```python
from build123d import *

# Parameters (mm, degrees)
SKETCH1_R           = 40
BOSS_EXTRUDE1_DEPTH = 100
SKETCH3_R           = 30
BOSS_EXTRUDE2_DEPTH = 180
SKETCH4_R           = 40
BOSS_EXTRUDE3_DEPTH = 100
SKETCH5_W           = 41.242816752
SKETCH5_H           = 81.516639277
CUT_EXTRUDE1_DEPTH  = 80
SKETCH6_W           = 41.962077935
SKETCH6_H           = 81.514478353
CUT_EXTRUDE2_DEPTH  = 80
FILLET3_R           = 40
FILLET4_R           = 40
SKETCH7_R           = 20
BOSS_EXTRUDE4_DEPTH = 10
SKETCH8_R           = 20
BOSS_EXTRUDE5_DEPTH = 10
FILLET5_R           = 40
FILLET6_R           = 40
FILLET7_R           = 10
FILLET8_R           = 10


# Some blends are built 0.0001 mm under size
with BuildPart() as part:
    # Sketch1 → Boss-Extrude1 (new body)
    with BuildSketch(Plane(origin=(0, 0, 0), x_dir=(1, 0, 0), z_dir=(0, 1, 0))):
        with Locations(Location((0, 0, 0), (0, 0, 270))):
            Circle(SKETCH1_R)
    extrude(amount=BOSS_EXTRUDE1_DEPTH)

    # Sketch3 → Boss-Extrude2 (add)
    with BuildSketch(Plane(origin=(0, 100, 0), x_dir=(1, 0, 0), z_dir=(0, 1, 0))):
        with Locations(Location((0, 0, 0), (0, 0, 90))):
            Circle(SKETCH3_R)
    extrude(amount=BOSS_EXTRUDE2_DEPTH)

    # Sketch4 → Boss-Extrude3 (add)
    with BuildSketch(Plane(origin=(0, 280, 0), x_dir=(1, 0, 0), z_dir=(0, 1, 0))):
        with Locations(Location((0, 0, 0), (0, 0, 270))):
            Circle(SKETCH4_R)
    extrude(amount=BOSS_EXTRUDE3_DEPTH)

    # Sketch5 → Cut-Extrude1 (cut)
    with BuildSketch(Plane(origin=(0, 380, 0), x_dir=(1, 0, 0), z_dir=(0, 1, 0))):
        with Locations((20.621408376, 0.242248556)):
            Rectangle(SKETCH5_W, SKETCH5_H)
    extrude(amount=-CUT_EXTRUDE1_DEPTH, mode=Mode.SUBTRACT)

    # Sketch6 → Cut-Extrude2 (cut)
    with BuildSketch(Plane.XZ):
        with Locations((20.981038968, -0.067313451)):
            Rectangle(SKETCH6_W, SKETCH6_H)
    extrude(amount=-CUT_EXTRUDE2_DEPTH, mode=Mode.SUBTRACT)

    # Fillet3
    fillet3_edges = [part.edges().sort_by_distance(p)[0] for p in [
        (-40, 0, 0),
    ]]
    fillet(fillet3_edges, radius=FILLET3_R - 0.0001)  # a hair under: the kernel refuses the full size

    # Fillet4
    fillet4_edges = [part.edges().sort_by_distance(p)[0] for p in [
        (-40, 380, 0),
    ]]
    fillet(fillet4_edges, radius=FILLET4_R - 0.0001)  # a hair under: the kernel refuses the full size

    # Sketch7 → Boss-Extrude4 (add)
    with BuildSketch(Plane(origin=(0, 0, 0), x_dir=(0, 0, -1), z_dir=(1, 0, 0))):
        with Locations(Location((0, 36.360995044, 0), (0, 0, 180))):
            Circle(SKETCH7_R)
    extrude(amount=BOSS_EXTRUDE4_DEPTH)

    # Sketch8 → Boss-Extrude5 (add)
    with BuildSketch(Plane(origin=(0, 0, 0), x_dir=(0, 0, -1), z_dir=(1, 0, 0))):
        with Locations(Location((0, 342.283138074, 0), (0, 0, 180))):
            Circle(SKETCH8_R)
    extrude(amount=BOSS_EXTRUDE5_DEPTH)

    # Fillet5
    # the kernel refuses this fillet: 40 mm, written as the material it adds along each edge
    with BuildSketch(Plane(origin=(0, 100, 0), x_dir=(0, 0, -1), z_dir=(1, 0, 0))) as fillet5_piece_1:
        with BuildLine():
            CenterArc((70, 26.457513111), FILLET5_R, 180, 41.409622109)
            Line((40, 0), (39.4, -0.529150262))
            ThreePointArc((39.4, -0.529150262), (35, -0.8), (30, -0.8))
            Line((30, -0.8), (29.2, 0))
            Line((29.2, 0), (29.2, 26.457513111))
            Line((29.2, 26.457513111), (30, 26.457513111))
        make_face()
    revolve(axis=Axis((0, 100, 0), (0, 1, 0)))

    # Fillet6
    # the kernel refuses this fillet: 40 mm, written as the material it adds along each edge
    with BuildSketch(Plane(origin=(0, 280, 0), x_dir=(0, 0, -1), z_dir=(1, 0, 0))) as fillet6_piece_1:
        with BuildLine():
            CenterArc((70, -26.457513111), FILLET6_R, 138.590377891, 41.409622109)
            Line((40, 0), (39.4, 0.529150262))
            ThreePointArc((39.4, 0.529150262), (35, 0.8), (30, 0.8))
            Line((30, 0.8), (29.2, 0))
            Line((29.2, 0), (29.2, -26.457513111))
            Line((29.2, -26.457513111), (30, -26.457513111))
        make_face()
    revolve(axis=Axis((0, 280, 0), (0, 1, 0)))

    # Fillet7
    fillet7_edges = [part.edges().sort_by_distance(p)[0] for p in [
        (40, 280, 0),
    ]]
    fillet(fillet7_edges, radius=FILLET7_R)

    # Fillet8
    fillet8_edges = [part.edges().sort_by_distance(p)[0] for p in [
        (-40, 100, 0),
    ]]
    fillet(fillet8_edges, radius=FILLET8_R)


solid = part.part
```
Build history of the part. All positions in model axes, mm. A direction names the side the tool comes from. Coordinates: 2 decimals unless noted, no trailing zeros. Order: outer loops, then holes, each group sorted by start corner. A loop starts at its lowest first (then second) coordinate and runs counter-clockwise, first axis right, second up. Notation, with made-up numbers: M 9.25,54 L 35.25,54 A19 ccw 35.25,66 Z; hole C 58.25,74.25 d8. An arc over 180 degrees is marked long. One line per question, with ' | ' between items. Start each with the question number.
1. Flat gauge pins, fed straight in: P1, Ø10, axis at y = 142.5, z = 10, coming from the -X side; P2, Ø1.5, axis at x = -5.5, y = 235, coming from the +Z side; P3, Ø1.5, axis at x = 15.5, z = -9, coming from the +Y side; P4, Ø6, axis at x = 30, z = -31, coming from the +Y side. Where does each tip first touch, or does it go through?
2. Wall check: line 1 along Y through (x, z) = (7, -12); line 2 along X through (y, z) = (277.5, 1.5); line 3 along Y through (x, z) = (-14.5, -30). Give the ranges that are in metal, low to high. Write a range as [from, to].
3. Cut at B-B (y = 113). Write the cut outline in (x, z).
4. Cut at A-A (y = 187.5). Write the cut outline in (x, z).
5. Tool access for faces 1 (the face through (10, 342, 0)), 2 (the face through (0, 323, -8)), 3 (the face through (15, 300, -1)), 4 (the face through (10, 36, 0)): list every direction of +Z, -Z, +X, -X, +Y, -Y with a clear straight run to the whole face (end or side of a thin tool).
The answers:
1) P1: stops at x = -29.58 | P2: stops at z = 29.62 | P3: stops at y = 300 | P4: passes through
2) line 1: y = [20.36, 52.36], [80, 300], [326.28, 358.28] | line 2: x = [-37.94, 37.94] | line 3: y = [17.87, 110.5], [269.5, 362.13]
3) outline: C 0,0 d64.66
4) outline: C 0,0 d60
5) face 1: +Z, -Z, +X, +Y | face 2: +X | face 3: +Z, -Z, +X | face 4: +Z, -Z, +X, -Y
